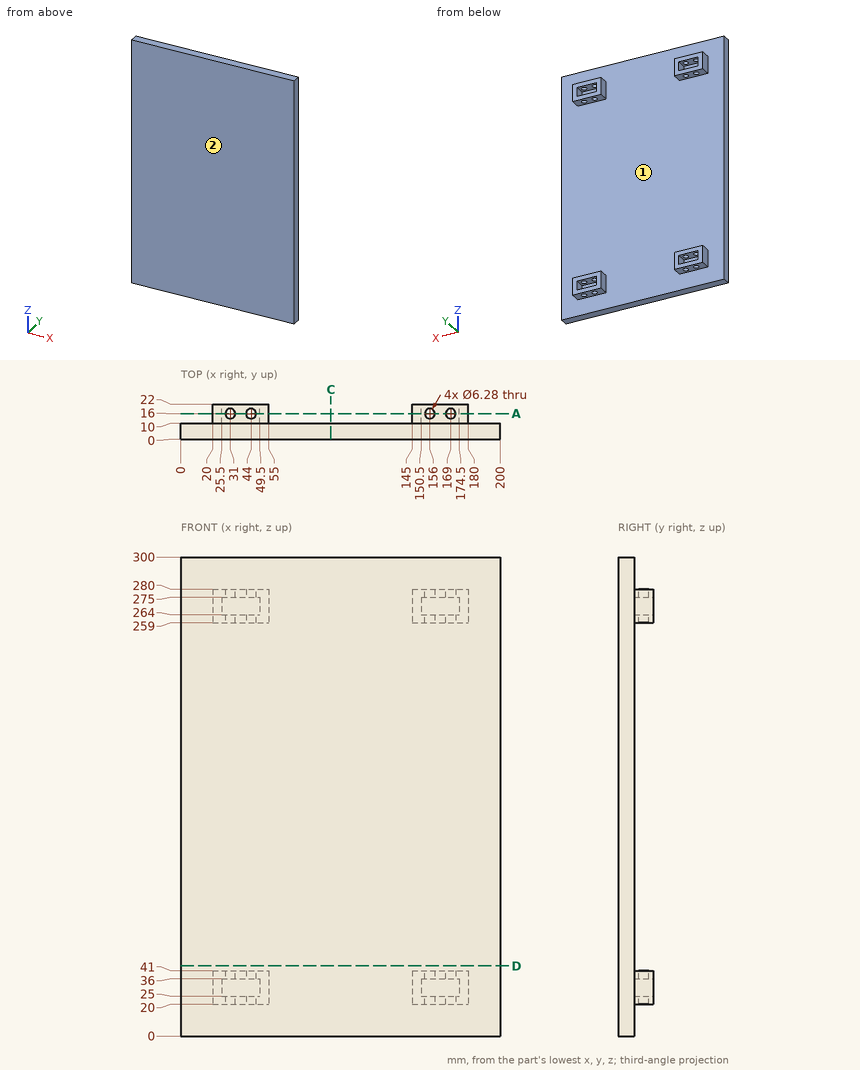
The drawing under review shows one solid part. Ordinate dimensions are in mm from its lowest x, y, z. Coordinates: 2 decimals unless noted, no trailing zeros. Write each loop counter-clockwise with the first axis right and the second up, starting at its lowest first coordinate (ties: lowest second). Pieces come first, ordered by that corner, then holes. Notation, with made-up numbers: M 39.5,39.5 L 56.5,39.5 A9 cw 56.5,49.5 Z; hole C -8.75,88 d5. An arc over 180 degrees is marked long. Answer as a JSON object with one key per item and string values.
Item 1: Insertion check: pin 1 Ø4 at (x, y) = (31, 16) entering from -Z; pin 2 Ø4 at (x, z) = (28, 129.5) entering from +Y; pin 3 Ø6 at (x, y) = (30.5, 15) entering from +Z; pin 4 Ø12 at (y, z) = (18, 30.5) entering from -X. Each pin has a flat end and moves straight along its axis. Give the tip position at first contact, or say it passes through.
Outcome:
{"pin 1": "through", "pin 2": "y = 10", "pin 3": "z = 280", "pin 4": "x = 20"}
Item 2: Add section D-D, the plane z = 44. Give the boundary of the cut face in (x, y), and give its area (3 significant figures).
Outcome:
{"outline": "M 0,0 L 200,0 L 200,10 L 0,10 Z", "area": "2,000 mm²"}
Item 3: Wall thickness on probe 1 along Z at (x, y) = (160, 20.5); probe 2 along Y at (x, z) = (169, 22.05); probe 3 along Z at (x, y) = (21.5, 17.75): over which ranges is each line inside the solid? List them lowest first.
Outcome:
{"probe 1": "20 to 25, 36 to 41, 259 to 264, 275 to 280", "probe 2": "0 to 12.86, 19.14 to 22", "probe 3": "20 to 41, 259 to 280"}
Item 4: Add section C-C, the plane x = 94. Give the boundary of the cut face in (y, z).
Outcome:
{"outline": "M 0,0 L 10,0 L 10,300 L 0,300 Z"}
Item 5: Add section A-A, the plane y = 16. State how many separate pieces and enclosed holes the cut face has, and give its area (3 significant figures).
Outcome:
{"separate pieces": "16", "enclosed holes": "0", "area": "1,380 mm²"}
Item 6: Draft analysis for pull direction Z (two halves, no side actions). For the marked faces 1 and 2, state which applies: pulls with the +Z half, pulls with the -Z half, needs draft (parallel to the pull), parting line crosses it, or undercut.
Outcome:
{"face 1": "undercut", "face 2": "needs draft"}
